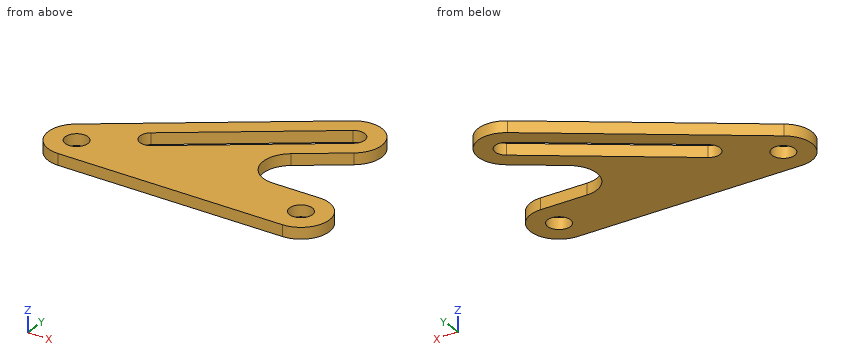
```python
from build123d import *

# Parameters (mm, degrees)
BOSS_EXTRUDE1_DEPTH     = 2
CUT_EXTRUDE1_DEPTH      = 4
CUT_EXTRUDE1_DEPTH_BACK = 107.639946795
SKETCH2_R               = 4
FILLET1_R               = 10


with BuildPart() as part:
    # Sketch1 → Boss-Extrude1 (new, symmetric)
    with BuildSketch(Plane.XY):
        with BuildLine():
            Line((61.625847103, 55.358628577), (-5.735764364, 8.191520443))
            ThreePointArc((-5.735764364, 8.191520443), (-3.007057995, 9.537169507), (0, 10))
            Line((0, 10), (31.715948024, 10))
            Line((31.715948024, 10), (73.09737583, 38.975587692))
            ThreePointArc((73.09737583, 38.975587692), (75.553131909, 52.902872498), (61.625847103, 55.358628577))
        make_face()
        with BuildLine():
            ThreePointArc((0, 10), (-3.007057995, 9.537169507), (-5.735764364, 8.191520443))
            ThreePointArc((-5.735764364, 8.191520443), (-9.537169507, -3.007057995), (0, -10))
            ThreePointArc((0, -10), (3.007057995, -9.537169507), (5.735764364, -8.191520443))
            Line((5.735764364, -8.191520443), (31.715948024, 10))
            Line((31.715948024, 10), (0, 10))
        make_face()
        with BuildLine():
            ThreePointArc((5.735764364, -8.191520443), (3.007057995, -9.537169507), (0, -10))
            Line((0, -10), (80, -10))
            ThreePointArc((80, -10), (90, 0), (80, 10))
            Line((80, 10), (31.715948024, 10))
            Line((31.715948024, 10), (5.735764364, -8.191520443))
        make_face()
    extrude(amount=BOSS_EXTRUDE1_DEPTH, both=True)

    # Sketch2 → Cut-Extrude1 (cut, two sides: drawn at the far end of the back side and taken through both)
    with BuildSketch(Plane.XY.offset(-CUT_EXTRUDE1_DEPTH_BACK)):
        Circle(SKETCH2_R)
        with Locations((80, 0)):
            Circle(SKETCH2_R)
        with BuildLine():
            Line((69.655917211, 43.890499957), (20.506794554, 9.475913776))
            ThreePointArc((20.506794554, 9.475913776), (14.935880632, 10.458216208), (15.918183063, 16.029130131))
            Line((15.918183063, 16.029130131), (65.067305721, 50.443716312))
            ThreePointArc((65.067305721, 50.443716312), (70.638219643, 49.46141388), (69.655917211, 43.890499957))
        make_face()
    extrude(amount=CUT_EXTRUDE1_DEPTH + CUT_EXTRUDE1_DEPTH_BACK, mode=Mode.SUBTRACT)

    # Fillet1
    fillet1_edges = [part.edges().sort_by_distance(p)[0] for p in [
        (31.715948024, 10, 0),
    ]]
    fillet(fillet1_edges, radius=FILLET1_R)


solid = part.part
```
Design review of the part built by this model. Coordinates are the model's own, in mm. Coordinates: 2 decimals unless noted, no trailing zeros. Loops run counter-clockwise (first coordinate to the right, second up) from the corner with the lowest first, then second, coordinate; pieces in that order, holes last. Notation, with made-up numbers: (-13.75, -28) - (35.25, -28) arc R12 cw to (35.25, -22) - close; hole circle Ø9 at (28.5, 82.25). An arc over 180 degrees is marked (long way). Use CSV: the item, a comma, the result in double quotes. Start each with the question number.
1) Consider section A-A on y = 0. Write out the cut boundary in (x, z).
2) Consider section D-D on y = 35.5. Write out the cut boundary in (x, z), then the cut area to 3 significant figures.
3) For pin 1 Ø1.5 at (y, z) = (40, -1) entering from -X; pin 2 Ø2 at (y, z) = (5, 1) entering from -X; pin 3 Ø1 at (y, z) = (27, 1) entering from +X, all flat-tipped, find the tip position at first contact; note any pin that passes through.
4) Consider section C-C on x = 23. Write out the cut boundary in (y, z), then the cut area to 3 significant figures.
5) Wall thickness on L1, parallel to X at y = 0, z = -1.05; L2, parallel to Y at x = 80, z = 0.1; L3, parallel to X at y = 29, z = 1.4: over which ranges is each line inside the solid? List them lowest first. Write a range as from..to.
6) Consider section B-B on z = 1.35. Write out the cut boundary in (x, y).
Geometry says:
1,outline,"(-10, -2) - (-4, -2) - (-4, 2) - (-10, 2) - close; (4, -2) - (76, -2) - (76, 2) - (4, 2) - close; (84, -2) - (90, -2) - (90, 2) - (84, 2) - close"
2,outline,"(33.26, -2) - (43.73, -2) - (43.73, 2) - (33.26, 2) - close; (57.67, -2) - (68.13, -2) - (68.13, 2) - (57.67, 2) - close"
2,area,"83.7 mm^2"
3,pin 1,"x = 38.62"
3,pin 2,"x = -9.17"
3,pin 3,"x = 56.82"
4,outline,"(-10, -2) - (11.22, -2) - (11.22, 2) - (-10, 2) - close; (20.99, -2) - (28.31, -2) - (28.31, 2) - (20.99, 2) - close"
4,area,"114 mm^2"
5,L1,"-10..-4, 4..76, 84..90"
5,L2,"-10..-4, 4..10"
5,L3,"23.98..34.44, 48.39..58.85"
6,outline,"(-5.74, 8.19) arc R10 ccw to (0, -10) - (80, -10) arc R10 ccw to (80, 10) - (63.43, 10) arc R10 cw to (57.7, 28.19) - (73.1, 38.98) arc R10 ccw to (61.63, 55.36) - close; hole circle Ø8 at (0, 0); hole (15.92, 16.03) arc R4 ccw to (20.51, 9.48) - (69.66, 43.89) arc R4 ccw to (65.07, 50.44) - close; hole circle Ø8 at (80, 0)"
